Input: part model. Units: mm. Frame: model coordinates. A direction names the side the tool comes from. Coordinates: 2 decimals unless noted, no trailing zeros. Loops run counter-clockwise (first coordinate to the right, second up) from the corner with the lowest first, then second, coordinate; pieces in that order, holes last. Notation, with made-up numbers: (52, -17.5) -> (78, -17.5) arc R16 ccw to (78, -9.5) -> close; hole circle Ø9 at (86, 79). An arc over 180 degrees is marked (long way). Answer as a JSON object with one key per item and string values.
from build123d import *

# Parameters (mm, degrees)
SKETCH1_W           = 60
SKETCH1_H           = 42
BOSS_EXTRUDE1_DEPTH = 8
SKETCH3_W           = 10
SKETCH3_H           = 42
BOSS_EXTRUDE5_DEPTH = 7
SKETCH5_W           = 14
SKETCH5_H           = 42
BOSS_EXTRUDE6_DEPTH = 11
SKETCH6_R           = 5
CUT_EXTRUDE1_DEPTH  = 75.759614766
FILLET1_R           = 7
FILLET2_R           = 5
FILLET3_R           = 5
BOSS_EXTRUDE7_DEPTH = 42


with BuildPart() as part:
    # Sketch1 → Boss-Extrude1 (new body)
    with BuildSketch(Plane(origin=(0, 0, 0), x_dir=(1, 0, 0), z_dir=(0, 1, 0))):
        with Locations((30, 21)):
            Rectangle(SKETCH1_W, SKETCH1_H)
    extrude(amount=BOSS_EXTRUDE1_DEPTH)

    # Sketch3 → Boss-Extrude5 (add)
    with BuildSketch(Plane(origin=(0, 8, 0), x_dir=(1, 0, 0), z_dir=(0, 1, 0))):
        with Locations((30, 21)):
            Rectangle(SKETCH3_W, SKETCH3_H)
    extrude(amount=BOSS_EXTRUDE5_DEPTH)

    # Sketch5 → Boss-Extrude6 (add)
    with BuildSketch(Plane.XZ):
        with Locations((30, -21)):
            Rectangle(SKETCH5_W, SKETCH5_H)
    extrude(amount=BOSS_EXTRUDE6_DEPTH)

    # Sketch6 → Cut-Extrude1 (cut, through all)
    with BuildSketch(Plane(origin=(0, 0, -42), x_dir=(-1, 0, 0), z_dir=(0, 0, -1))):
        with Locations((-30, -5)):
            Circle(SKETCH6_R)
    extrude(amount=-CUT_EXTRUDE1_DEPTH, mode=Mode.SUBTRACT)

    # Fillet1
    fillet1_edges = [part.edges().sort_by_distance(p)[0] for p in [
        (23, -11, -21),
        (37, -11, -21),
    ]]
    fillet(fillet1_edges, radius=FILLET1_R - 0.0001)  # a hair under: the kernel refuses the full size

    # Fillet2
    fillet2_edges = [part.edges().sort_by_distance(p)[0] for p in [
        (23, 0, -21),
    ]]
    fillet(fillet2_edges, radius=FILLET2_R)

    # Fillet3
    fillet3_edges = [part.edges().sort_by_distance(p)[0] for p in [
        (37, 0, -21),
    ]]
    fillet(fillet3_edges, radius=FILLET3_R)

    # Sketch8 → Boss-Extrude7 (add)
    with BuildSketch(Plane(origin=(0, 0, -42), x_dir=(-1, 0, 0), z_dir=(0, 0, -1))):
        with BuildLine():
            Line((-41.958260743, -1), (-42.958260743, 0))
            Line((-42.958260743, 0), (-41.958260743, 0))
            ThreePointArc((-41.958260743, 0), (-38.573244741, -1.320099639), (-36.9756521, -4.583333333))
            ThreePointArc((-36.9756521, -4.583333333), (-34.739022403, -9.151860505), (-30, -11))
            ThreePointArc((-30, -11), (-25.260977597, -9.151860505), (-23.0243479, -4.583333333))
            ThreePointArc((-23.0243479, -4.583333333), (-21.426755259, -1.320099639), (-18.041739257, 0))
            Line((-18.041739257, 0), (-16.803044796, 0))
            Line((-16.803044796, 0), (-18.041739257, -1))
            ThreePointArc((-18.041739257, -1), (-20.749752058, -2.056079711), (-22.027826171, -4.666666667))
            ThreePointArc((-22.027826171, -4.666666667), (-24.583974397, -9.887840578), (-30, -12))
            ThreePointArc((-30, -12), (-35.416025603, -9.887840578), (-37.972173829, -4.666666667))
            ThreePointArc((-37.972173829, -4.666666667), (-39.250247942, -2.056079711), (-41.958260743, -1))
        make_face()
    extrude(amount=-BOSS_EXTRUDE7_DEPTH)


solid = part.part
1. Section query A-A (z = -27). Return loops of the section in (x, y).
Reply:
{"outline": "(0, 0) -> (16.8, 0) -> (18.04, -1) arc R4 cw to (22.03, -4.67) arc R8 ccw to (37.97, -4.67) arc R4 cw to (41.96, -1) -> (42.96, 0) -> (60, 0) -> (60, 8) -> (35, 8) -> (35, 15) -> (25, 15) -> (25, 8) -> (0, 8) -> close; hole circle Ø10 at (30, -5)"}
2. Section query B-B (y = -6.25). Return loops of the section in (x, z), plus the area to 3 significant figures.
Reply:
{"outline": "(22.32, -42) -> (25.16, -42) -> (25.16, 0) -> (22.32, 0) -> close; (34.84, -42) -> (37.68, -42) -> (37.68, 0) -> (34.84, 0) -> close", "area": "238 mm2"}
3. Mould query, pull axis Y, two halves, no side actions, for faces 1 (the face through (17.41, -0.49, -21.29)), 2 (the face through (30, 5, -42)), 3 (the face through (35, -5, -21)). Classes: pulls with the +Y half, pulls with the -Y half, needs draft (parallel to the pull), parting line crosses it, or undercut.
Reply:
{"face 1": "pulls with the -Y half", "face 2": "needs draft", "face 3": "undercut"}
4. Line query: line 1 along Y through (x, z) = (30, -27); line 2 along X through (y, z) = (14.25, -4); line 3 along X through (y, z) = (-9.5, -15.5). Output: solid intervals per line, ascending.
Reply:
{"line 1": "y = -12 to -10, 0 to 15", "line 2": "x = 25 to 35", "line 3": "x = 24.19 to 27.82, 32.18 to 35.81"}
5. Section query D-D (y = -2.5). Return loops of the section in (x, z), plus the area to 3 significant figures.
Reply:
{"outline": "(21.16, -42) -> (25.67, -42) -> (25.67, 0) -> (21.16, 0) -> close; (34.33, -42) -> (38.84, -42) -> (38.84, 0) -> (34.33, 0) -> close", "area": "378 mm2"}
6. Access query for faces 4 (the face through (51, 0, -21)), 5 (the face through (25, 11, -21)), 6 (the face through (8, 0, -21)), 7 (the face through (30, 5, 0)), 8 (the face through (47, 8, -21)). Directions: +Z, -Z, +X, -X, +Y, -Y. A direction counts if a zero-diameter tool reaches every point of the face in a straight line with its end or side. Return the directions, or none.
Reply:
{"face 4": "+Z, -Z, +X, -Y", "face 5": "+Z, -Z, -X, +Y", "face 6": "+Z, -Z, -X, -Y", "face 7": "+Z, +X, -X, +Y, -Y", "face 8": "+Z, -Z, +X, +Y"}
7. Pin query (flat end, axial travel): P1, Ø5, axis at y = -5, z = -34.5, coming from the +X side; P2, Ø3, axis at x = 36.5, z = -31.5, coming from the -Y side (3 decimals); P3, Ø5, axis at x = 53, z = -27, coming from the -Y side. Return the tip coordinate at first contact, or that it passes through.
Reply:
{"P1": "stops at x = 38.84", "P2": "stops at y = -10.245", "P3": "stops at y = 0"}
8. Section query C-C (x = 5). Return loops of the section in (y, z).
Reply:
{"outline": "(0, -42) -> (8, -42) -> (8, 0) -> (0, 0) -> close"}
